```python
from build123d import *

# Parameters (mm, degrees)
SKETCH_1_R           = 41
SKETCH_1_R_2         = 39
EXTRUDE_1_DEPTH      = 20
EXTRUDE_START        = -14
EXTRUDE_2_DEPTH      = 14
EXTRUDE_START_2      = -3
SKETCH_3_R           = 4
SKETCH_3_R_2         = 1
EXTRUDE_3_DEPTH      = 3
CUT_EXTRUDE_3_DEPTH  = 3
EXTRUDE_5_DEPTH      = 10
EXTRUDE_5_DEPTH_BACK = 15
SKETCH_1_2_R         = 41
SKETCH_1_2_R_2       = 39
EXTRUDE_START_3      = 10
EXTRUDE_7_DEPTH      = 10
EXTRUDE_8_DEPTH      = 10
EXTRUDE_8_DEPTH_BACK = 5
CUT_EXTRUDE_4_DEPTH  = 10
EXTRUDE_9_DEPTH      = 10
EXTRUDE_9_DEPTH_BACK = 1.5
CUT_EXTRUDE_6_DEPTH  = 10
SKETCH_16_R          = 1.22
CUT_EXTRUDE_7_DEPTH  = 3


with BuildPart() as part:
    # Sketch 1 → Extrude 1 (new body)
    with BuildSketch(Plane(origin=(0, 0, 0), x_dir=(1, 0, 0), z_dir=(0, 1, 0))):
        with Locations(Location((0, 0, 0), (0, 0, 270))):
            Circle(SKETCH_1_R)
        with Locations(Location((0, 0, 0), (0, 0, 270))):
            Circle(SKETCH_1_R_2, mode=Mode.SUBTRACT)
    extrude(amount=EXTRUDE_1_DEPTH)

    # Sketch 2 → Extrude 2 (add)
    with BuildSketch(Plane(origin=(0, 20, 0), x_dir=(1, 0, 0), z_dir=(0, 1, 0)).offset(EXTRUDE_START)):
        with BuildLine():
            Line((-20, -41), (3.5e-08, -41))
            ThreePointArc((3.5e-08, -41), (-10.333598732, -39.676400256), (-20, -35.791060336))
            Line((-20, -35.791060336), (-20, -41))
        make_face()
        with BuildLine():
            Line((3.5e-08, -41), (20, -41))
            Line((20, -41), (20, -35.791060336))
            ThreePointArc((20, -35.791060336), (10.333598766, -39.676400247), (3.5e-08, -41))
        make_face()
    extrude(amount=EXTRUDE_2_DEPTH)

    # Sketch 3 → Extrude 3 (add)
    with BuildSketch(Plane(origin=(0, 20, 0), x_dir=(1, 0, 0), z_dir=(0, 1, 0)).offset(EXTRUDE_START_2)):
        with BuildLine():
            Line((-2, 38.948684188), (-2, 8.774964387))
            ThreePointArc((-2, 8.774964387), (-7.794228634, 4.5), (-8.599342077, -2.655431386))
            Line((-8.599342077, -2.655431386), (-34.730549951, -17.742291287))
            ThreePointArc((-34.730549951, -17.742291287), (-33.774990748, -19.5), (-32.730549951, -21.206392902))
            Line((-32.730549951, -21.206392902), (-6.599342077, -6.119533001))
            ThreePointArc((-6.599342077, -6.119533001), (0, -9), (6.599342077, -6.119533001))
            Line((6.599342077, -6.119533001), (32.730549951, -21.206392902))
            ThreePointArc((32.730549951, -21.206392902), (33.774990748, -19.5), (34.730549951, -17.742291287))
            Line((34.730549951, -17.742291287), (8.599342077, -2.655431386))
            ThreePointArc((8.599342077, -2.655431386), (7.794228634, 4.5), (2, 8.774964387))
            Line((2, 8.774964387), (2, 38.948684188))
            ThreePointArc((2, 38.948684188), (0, 39), (-2, 38.948684188))
        make_face()
        with Locations(Location((0, 0, 0), (0, 0, 270))):
            Circle(SKETCH_3_R, mode=Mode.SUBTRACT)
        with Locations(Location((-6, 0, 0), (0, 0, 270))):
            Circle(SKETCH_3_R_2, mode=Mode.SUBTRACT)
        with Locations(Location((6, 0, 0), (0, 0, 270))):
            Circle(SKETCH_3_R_2, mode=Mode.SUBTRACT)
    extrude(amount=EXTRUDE_3_DEPTH)

    # Sketch 7 → Cut-Extrude 3 (cut)
    with BuildSketch(Plane.XZ.offset(-6)):
        with BuildLine():
            Line((0, 41), (-20, 41))
            Line((-20, 41), (-20, 35.791060336))
            ThreePointArc((-20, 35.791060336), (-10.333598749, 39.676400251), (0, 41))
        make_face()
        with BuildLine():
            Line((20, 41), (0, 41))
            ThreePointArc((0, 41), (10.333598749, 39.676400251), (20, 35.791060336))
            Line((20, 35.791060336), (20, 41))
        make_face()
    extrude(amount=-CUT_EXTRUDE_3_DEPTH, mode=Mode.SUBTRACT)

    # Sketch 1_2 → Extrude 5 (add, two sides: drawn at the far end of the back side and taken through both)
    with BuildSketch(Plane(origin=(0, 0, 0), x_dir=(1, 0, 0), z_dir=(0, 1, 0)).offset(-EXTRUDE_5_DEPTH_BACK)):
        with Locations(Location((0, 0, 0), (0, 0, 270))):
            Circle(SKETCH_1_2_R)
        with Locations(Location((0, 0, 0), (0, 0, 92.939534486))):
            Circle(SKETCH_1_2_R_2, mode=Mode.SUBTRACT)
    extrude(amount=EXTRUDE_5_DEPTH + EXTRUDE_5_DEPTH_BACK)

    # Sketch 7_4 → Extrude 7 (add)
    with BuildSketch(Plane.XZ.offset(-6).offset(EXTRUDE_START_3)):
        with BuildLine():
            Line((0, 41), (-20, 41))
            Line((-20, 41), (-20, 35.791060336))
            ThreePointArc((-20, 35.791060336), (-10.333598749, 39.676400251), (0, 41))
        make_face()
        with BuildLine():
            Line((20, 41), (0, 41))
            ThreePointArc((0, 41), (10.333598749, 39.676400251), (20, 35.791060336))
            Line((20, 35.791060336), (20, 41))
        make_face()
    extrude(amount=-EXTRUDE_7_DEPTH)

    # Sketch 7_5 → Extrude 8 (add, two sides: drawn at the far end of the back side and taken through both)
    with BuildSketch(Plane.XZ.offset(-6).offset(-EXTRUDE_8_DEPTH_BACK)):
        with BuildLine():
            Line((0, 41), (-20, 41))
            Line((-20, 41), (-20, 35.791060336))
            ThreePointArc((-20, 35.791060336), (-10.333598749, 39.676400251), (0, 41))
        make_face()
        with BuildLine():
            Line((20, 41), (0, 41))
            ThreePointArc((0, 41), (10.333598749, 39.676400251), (20, 35.791060336))
            Line((20, 35.791060336), (20, 41))
        make_face()
    extrude(amount=EXTRUDE_8_DEPTH + EXTRUDE_8_DEPTH_BACK)

    # Sketch 4 → Cut-Extrude 4 (cut)
    with BuildSketch(Plane.XY.offset(41)):
        Polygon((-10, 4.766838493), (-7.2, 6.383419246), (-7.2, 9.616580754), (-10, 11.233161507), (-12.8, 9.616580754), (-12.8, 6.383419246), align=None)
        Polygon((12.8, 6.383419246), (10, 4.766838493), (7.2, 6.383419246), (7.2, 9.616580754), (10, 11.233161507), (12.8, 9.616580754), align=None)
    extrude(amount=-CUT_EXTRUDE_4_DEPTH, mode=Mode.SUBTRACT)

    # Sketch 4_3 → Extrude 9 (add, two sides: drawn at the far end of the back side and taken through both)
    with BuildSketch(Plane.XY.offset(41).offset(-EXTRUDE_9_DEPTH_BACK)):
        Polygon((-10, 4.766838493), (-7.2, 6.383419246), (-7.2, 9.616580754), (-10, 11.233161507), (-12.8, 9.616580754), (-12.8, 6.383419246), align=None)
        Polygon((12.8, 6.383419246), (10, 4.766838493), (7.2, 6.383419246), (7.2, 9.616580754), (10, 11.233161507), (12.8, 9.616580754), align=None)
    extrude(amount=EXTRUDE_9_DEPTH + EXTRUDE_9_DEPTH_BACK)

    # Sketch 13 → Cut-Extrude 6 (cut)
    with BuildSketch(Plane.XY.offset(51)):
        Polygon((10, 11.233161507), (7.2, 9.616580754), (7.2, 6.383419246), (10, 4.766838493), (12.8, 6.383419246), (12.8, 9.616580754), align=None)
        Polygon((-10, 11.233161507), (-12.8, 9.616580754), (-12.8, 6.383419246), (-10, 4.766838493), (-7.2, 6.383419246), (-7.2, 9.616580754), align=None)
    extrude(amount=-CUT_EXTRUDE_6_DEPTH, mode=Mode.SUBTRACT)

    # Sketch 16 → Cut-Extrude 7 (cut)
    with BuildSketch(Plane.XY.offset(41)):
        with Locations((-10, 8)):
            Circle(SKETCH_16_R)
        with Locations(Location((10, 8, 0), (0, 0, 180))):
            Circle(SKETCH_16_R)
    extrude(amount=-CUT_EXTRUDE_7_DEPTH, mode=Mode.SUBTRACT)


solid = part.part
```
Verification items for the finished model (mm, model axes). A direction names the side the tool comes from. Round coordinates to 2 decimals unless told otherwise and drop trailing zeros. Write each loop counter-clockwise with the first axis right and the second up, starting at its lowest first coordinate (ties: lowest second). Pieces come first, ordered by that corner, then holes.
1. Access from +Z, -Z, +X, -X, +Y, -Y to the whole of each face (thin tool, end or side, straight path). Record for faces 1 (the flat face through (19.482, 18.479, 13.557)), 2 (the flat face through (0, 8, 41)), 3 (the flat face through (15, -4, 39)), 4 (the flat face through (10, 6.6, 39.5)).
2. Scan lines: L1, parallel to X at y = 6, z = 0; L2, parallel to Z at x = -24.5, y = 8; L3, parallel to Z at x = 4, y = 3.5. Record each from-to range of solid material in increasing order.
3. Section check D-D on y = -13. Enter the section's corners in (x, z), plus the area to 3 significant figures.
4. Section check A-A on z = 0. Enter the section's corners in (x, y), plus the area to 3 significant figures.
5. Section check B-B on y = 13. Enter the section's corners in (x, z).
6. Draft check along X on faces 5 (the flat face through (20, 8, 38)), 6 (the flat face through (-15, -4, 40)), 7 (the flat face through (-0.2, 17, 4.3)). Enter one of: +X half, -X half, draft (parallel to the pull), parting line (faces both ways), or undercut.
7. Gauge pin test, flat ends, axial feed: P1, Ø1.5, axis at y = 19, z = -18, coming from the -X side; P2, Ø3, axis at x = 24, y = -3, coming from the +Z side; P3, Ø3, axis at x = 9.5, y = 7, coming from the -Z side; P4, Ø4, axis at x = 5, z = 38, coming from the -Y side. Record the tip position at first contact, or that the pin passes through.
8. Section check C-C on x = -24. Enter the section's corners in (y, z), plus the area to 3 significant figures.
Answer:
1. face 1: +Y, -Y
1. face 2: +Z, +X, -X, +Y, -Y
1. face 3: +Z, +X, -Y
1. face 4: none
2. L1: x = -41 to -39, 39 to 41
2. L2: z = -32.87 to -30.34, 30.34 to 32.87
2. L3: z = -40.8 to -38.79, 38.79 to 41
3. outline: circle Ø82 at (0, 0); hole circle Ø78 at (0, 0)
3. area: 503 mm2
4. outline: (-41, -15) - (-39, -15) - (-39, 20) - (-41, 20) - close; (-9, 17) - (-7, 17) - (-7, 20) - (-9, 20) - close; (-5, 17) - (-4, 17) - (-4, 20) - (-5, 20) - close; (4, 17) - (5, 17) - (5, 20) - (4, 20) - close; (7, 17) - (9, 17) - (9, 20) - (7, 20) - close; (39, -15) - (41, -15) - (41, 20) - (39, 20) - close
4. area: 158 mm2
5. outline: (-20, 35.79) arc R41 ccw (long way) to (20, 35.79) - (20, 41) - (-20, 41) - close; hole circle Ø78 at (0, 0)
6. face 5: +X half
6. face 6: draft
6. face 7: undercut
7. P1: stops at x = -37.19
7. P2: stops at z = 34.27
7. P3: stops at z = -40.21
7. P4: stops at y = -15
8. outline: (-15, -33.24) - (20, -33.24) - (20, -30.74) - (-15, -30.74) - close; (-15, 30.74) - (20, 30.74) - (20, 33.24) - (-15, 33.24) - close; (17, 11.55) - (20, 11.55) - (20, 16.17) - (17, 16.17) - close
8. area: 189 mm2
